Design review of the part built by this model. Coordinates are the model's own, in mm. Face numbers are marked on the shaded views. A direction names the side the tool comes from. Round coordinates to 2 decimals unless told otherwise and drop trailing zeros. Order: outer loops, then holes, each group sorted by start corner. A loop starts at its lowest first (then second) coordinate and runs counter-clockwise, first axis right, second up. Notation, with made-up numbers: M -26.75,88.5 L 25.25,88.5 A29 ccw 25.25,127.5 Z; hole C -14,21 d6. An arc over 180 degrees is marked long. Use a Markdown table: item, result. Add a question column.
(1) Take a section at D-D (x = 20.5). Write out the cut boundary in (y, z), then the cut area to 3 significant figures.
(2) Take a section at A-A (y = 0). Write out the cut boundary in (x, z), then the cut area to 3 significant figures.
(3) Take a section at C-C (x = -13.5). Write out the cut boundary in (y, z), then the cut area to 3 significant figures.
(4) Take a section at B-B (z = 3). Write out the cut boundary in (x, y).
(5) For pin 1 (8 mm diameter, centred on x = -12.11, y = -39.46, fed in from +Z); pin 2 (15 mm diameter, centred on x = -10.5, z = 30.5, fed in from -Y); pin 3 (5 mm diameter, centred on x = -7.5, y = 34, fed in from +Z); pin 4 (1 mm diameter, centred on x = -7, y = 8.5, fed in from +Z), all flat-tipped, find the tip position at first contact; note any pin that passes through.
(6) To check wall thickness, follow probe 1 along X at (y, z) = (46, 30); probe 2 along Y at (x, z) = (7.5, 7.5); probe 3 along Y at (x, z) = (-13.5, 10). State the ranges of each line that lie inside material, in increasing order. Write a range as from..to.
(7) Machinability: for the marked faces 5, 6, 7, 8 and 9, which of the approach directions +Z, -Z, +X, -X, +Y, -Y give a long, thin tool a straight path to every point of the face, cutting with its end or side? Answer none if there is none.
(8) The part is to be moulded in two halves that separate along Y. For the marked faces 1, 2, 3 and 4, say which applies: released by +Y, released by -Y, zero draft, split by the parting line, or undercut.
```python
from build123d import *

# Parameters (mm, degrees)
F0_W     = 11
F0_H     = 11
F0_H_2   = 30
F1_DEPTH = 24
F3_DEPTH = 12.5
F4_R     = 2.5
F4_R_2   = 5
F5_DEPTH = 56
F6_R     = 13
F7_R     = 5
F8_R     = 5


with BuildPart() as f1:
    # F0 (on Right) → F1 (new body, symmetric)
    with BuildSketch(Plane.YZ):
        with BuildLine():
            Line((-51, 0), (-30, 0))
            ThreePointArc((-30, 0), (-29.4730143031, 5.5983415304), (-27.9105714739, 11))
            Line((-27.9105714739, 11), (-51, 11))
            Line((-51, 11), (-51, 0))
        make_face()
        with BuildLine():
            ThreePointArc((-27.9105714739, 11), (-29.4730143031, 5.5983415304), (-30, 0))
            Line((-30, 0), (-19, 0))
            ThreePointArc((-19, 0), (-18.1017503893, 5.7729223833), (-15.4919333848, 11))
            Line((-15.4919333848, 11), (-27.9105714739, 11))
        make_face()
        with BuildLine():
            Line((15.4919333848, 11), (27.9105714739, 11))
            ThreePointArc((27.9105714739, 11), (0, 30), (-27.9105714739, 11))
            Line((-27.9105714739, 11), (-15.4919333848, 11))
            ThreePointArc((-15.4919333848, 11), (0, 19), (15.4919333848, 11))
        make_face()
        with BuildLine():
            Line((19, 0), (30, 0))
            ThreePointArc((30, 0), (29.4730143031, 5.5983415304), (27.9105714739, 11))
            Line((27.9105714739, 11), (15.4919333848, 11))
            ThreePointArc((15.4919333848, 11), (18.1017503893, 5.7729223833), (19, 0))
        make_face()
        with BuildLine():
            ThreePointArc((27.9105714739, 11), (29.4730143031, 5.5983415304), (30, 0))
            Line((30, 0), (45, 0))
            Line((45, 0), (45, 11))
            Line((45, 11), (27.9105714739, 11))
        make_face()
        with Locations((50.5, 5.5)):
            Rectangle(F0_W, F0_H)
        with Locations((50.5, 26)):
            Rectangle(F0_W, F0_H_2)
    extrude(amount=F1_DEPTH, both=True)

    # F2 (on face) → F3 (cut, symmetric)
    with BuildSketch(Plane(origin=(0, 56, 0), x_dir=(-1, 0, 0), z_dir=(0, 1, 0))):
        with BuildLine():
            ThreePointArc((-6.5, 25), (0, 18.5), (6.5, 25))
            ThreePointArc((6.5, 25), (0, 31.5), (-6.5, 25))
        make_face()
        with BuildLine():
            ThreePointArc((-6.5, 25), (0, 31.5), (6.5, 25))
            Line((6.5, 25), (6.5, 41))
            Line((6.5, 41), (-6.5, 41))
            Line((-6.5, 41), (-6.5, 25))
        make_face()
    extrude(amount=F3_DEPTH, both=True, mode=Mode.SUBTRACT)

    # F4 (on Top) → F5 (cut, symmetric)
    with BuildSketch(Plane.XY):
        Circle(F4_R)
        with Locations((-12.1131800115, -39.455285737)):
            Circle(F4_R_2)
        with Locations((9.8868199885, -39.455285737)):
            Circle(F4_R_2)
    extrude(amount=F5_DEPTH, both=True, mode=Mode.SUBTRACT)

    # F6
    f6_edges = [f1.edges().sort_by_distance(p)[0] for p in [
        (-24, -51, 5.5),
        (24, -51, 5.5),
    ]]
    fillet(f6_edges, radius=F6_R)

    # F7
    f7_edges = [f1.edges().sort_by_distance(p)[0] for p in [
        (-24, 50.5, 41),
        (24, 50.5, 41),
    ]]
    fillet(f7_edges, radius=F7_R)

    # F8
    f8_edges = [f1.edges().sort_by_distance(p)[0] for p in [
        (0, 27.910571, 11),
        (0, -27.910571, 11),
    ]]
    fillet(f8_edges, radius=F8_R)


solid = f1.part
```
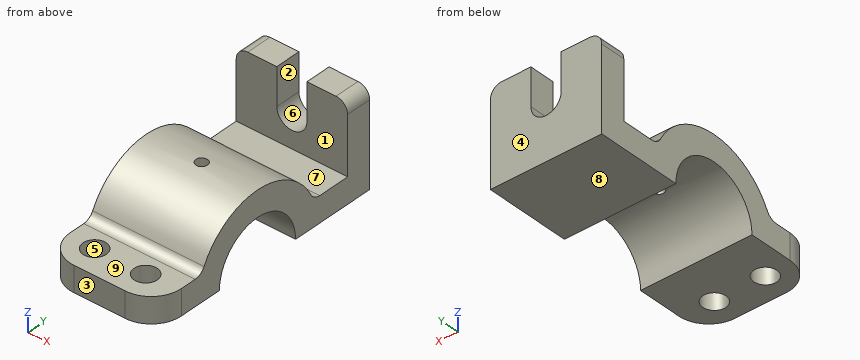
Verdict:
| question | item | result |
|---|---|---|
| 1 | outline | M -46.87,0 L -19,0 A19 cw 19,0 L 56,0 L 56,40.77 L 45,40.77 L 45,11 L 31.13,11 A5 cw 26.68,13.71 A30 ccw -26.68,13.71 A5 cw -31.13,11 L -46.87,11 Z |
| 1 | area | 1,660 mm^2 |
| 2 | outline | M -24,19 L -2.5,19 L -2.5,30 L -24,30 Z; M 2.5,19 L 24,19 L 24,30 L 2.5,30 Z |
| 2 | area | 473 mm^2 |
| 3 | outline | M -50.76,0 L -44.26,0 L -44.26,11 L -50.76,11 Z; M -34.65,0 L -19,0 A19 cw 19,0 L 56,0 L 56,41 L 45,41 L 45,11 L 31.13,11 A5 cw 26.68,13.71 A30 ccw -26.68,13.71 A5 cw -31.13,11 L -34.65,11 Z |
| 3 | area | 1,600 mm^2 |
| 4 | outline | M -24,-38 A13 ccw -11,-51 L 11,-51 A13 ccw 24,-38 L 24,-18.76 L -24,-18.76 Z; M -24,18.76 L 24,18.76 L 24,56 L -24,56 Z; hole C -12.11,-39.46 d10; hole C 9.89,-39.46 d10 |
| 5 | pin 1 | passes through |
| 5 | pin 2 | stops at y = -19.26 |
| 5 | pin 3 | stops at z = 11 |
| 5 | pin 4 | stops at z = 28.91 |
| 6 | probe 1 | x = -24..-6.5, 6.5..24 |
| 6 | probe 2 | y = -51..-43.85, -35.06..-17.46, 17.46..56 |
| 6 | probe 3 | y = -50.76..-44.26, -34.65..-16.16, 16.16..56 |
| 7 | face 5 | +Z, -Z |
| 7 | face 6 | +Z, +Y |
| 7 | face 7 | +Z, +X, -X |
| 7 | face 8 | -Z, +X, -X, +Y, -Y |
| 7 | face 9 | +Z, +X, -X, -Y |
| 8 | face 1 | undercut |
| 8 | face 2 | zero draft |
| 8 | face 3 | released by -Y |
| 8 | face 4 | released by +Y |
